Geometry: final body of the model. Coordinates: model frame, mm. A direction names the side the tool comes from. Give positions to 0.01 mm unless a question says otherwise; leave off trailing zeros. Write each loop counter-clockwise with the first axis right and the second up, starting at its lowest first coordinate (ties: lowest second). Pieces come first, ordered by that corner, then holes. Notation, with made-up numbers: (-37, 58) -> (-10, 58) arc R25 ccw to (-10, 82) -> close; hole circle Ø8 at (25.25, -16). An arc over 180 degrees is marked (long way). Answer in a Markdown table with one row per item. Add a question column.
Item 1: Section query B-B on x = 14.5. Output: boundary loops of the cut face in (y, z), plus the area to 3 significant figures.
Item 2: Material intervals for probe 1 along Z at (x, y) = (-37, 23.5); probe 2 along X at (y, z) = (1, 5.5); probe 3 along Y at (x, z) = (-21, 5.5), sorted ascending. Write a range as from..to.
Item 3: Access query for faces 1 (the flat face through (-56.448, 10, 1)), 2 (the cylindrical face through (54.28, 10.45, 8.57)). Directions: +Z, -Z, +X, -X, +Y, -Y. A direction counts if a zero-diameter tool reaches every point of the face in a straight line with its end or side. Return the directions, or none.
Item 4: First-contact query: P1, Ø8, axis at x = -18.5, y = 3.5, coming from the -Z side; P2, Ø4, axis at y = -0.5, z = 8, coming from the +X side; P3, Ø4, axis at y = 14, z = 2, coming from the -X side. Flat tips, straight axial feed; report the tip coordinate or a pass-through.
```python
from build123d import *

# Parameters (mm, degrees)
F0_W     = 120
F0_H     = 41.8604637527
F1_DEPTH = 10
F2_W     = 112.2293550894
F2_H     = 2.9544678982
F3_DEPTH = 73.9
F4_R     = 4.99999


# Not quite as in the source:
# - a fillet or chamfer is up to 0.001 mm smaller than in the source, because OpenCascade refuses the exact size


with BuildPart() as f1:
    # F0 (on Top) → F1 (new body)
    with BuildSketch(Plane.XY):
        with Locations((-4.2187506333, 10.1562498603)):
            Rectangle(F0_W, F0_H)
    extrude(amount=F1_DEPTH)

    # F2 (on face) → F3 (cut)
    with BuildSketch(Plane.XZ.offset(10.773982016)):
        with Locations((-0.333428178, 1.4772339491)):
            Rectangle(F2_W, F2_H)
    extrude(amount=-F3_DEPTH, mode=Mode.SUBTRACT)

    # F4 (radius 5 in the source; OpenCascade refuses exactly that, so slightly less here)
    f4_edges = [f1.edges().sort_by_distance(p)[0] for p in [
        (-64.218751, 10.15625, 10),
        (-4.218751, 31.086482, 10),
        (-4.218751, -10.773982, 10),
        (55.781249, 10.15625, 10),
        (-64.218751, 10.15625, 0),
    ]]
    fillet(f4_edges, radius=F4_R)


solid = f1.part
```
Findings below:
| question | item | result |
|---|---|---|
| 1 | outline | (-10.77, 2.95) -> (31.09, 2.95) -> (31.09, 5) arc R5 ccw to (26.09, 10) -> (-5.77, 10) arc R5 ccw to (-10.77, 5) -> close |
| 1 | area | 284 mm^2 |
| 2 | probe 1 | z = 2.95..10 |
| 2 | probe 2 | x = -64.19..55.76 |
| 2 | probe 3 | y = -10.75..31.06 |
| 3 | face 1 | -Z, +X, +Y, -Y |
| 3 | face 2 | +Z, +X, +Y, -Y |
| 4 | P1 | stops at z = 2.95 |
| 4 | P2 | stops at x = 55.68 |
| 4 | P3 | stops at x = -64.12 |
